Here's how the part is built. I have some questions about the finished solid (model axes, mm). Face numbers are marked on the shaded views. A direction names the side the tool comes from. Round coordinates to 2 decimals unless told otherwise and drop trailing zeros. Write each loop counter-clockwise with the first axis right and the second up, starting at its lowest first coordinate (ties: lowest second). Pieces come first, ordered by that corner, then holes. Notation, with made-up numbers: (69, 78.25) -> (89, 78.25) arc R28 cw to (89, 101.25) -> close; hole circle Ø4 at (-2, 20.25). An arc over 180 degrees is marked (long way). Put each result on its own line as item: value. Start each with the question number.
1. I need wall thicknesses on probe 1 along X at (y, z) = (5.75, 13); probe 2 along Z at (x, y) = (38.5, -3.75); probe 3 along Y at (x, z) = (0, 18.75). Which ranges of each line are inside material? Lowest first, please. Write a range as from..to.
2. We'd pull the mould along X, two halves only. Please class the marked faces 6, 7 and 8: +X half, -X half, draft (parallel to the pull), parting line (faces both ways), or undercut.
3. Which directions (+Z, -Z, +X, -X, +Y, -Y) give clear straight access to the entire face, cutting with the end or side of a thin tool? Please do the marked faces 1, 2, 3, 4 and 5.
4. Suppose I cut it at D-D (z = 6). Please give me the cut outline in (x, y), then the cut area to 3 significant figures.
5. Suppose I cut it at B-B (x = 38.5). Please give me the cut outline in (y, z), then the cut area to 3 significant figures.
6. For pin 1 (3 mm diameter, centred on y = 40, z = 13.5, fed in from +X); pin 2 (6 mm diameter, centred on x = -27.5, y = 18.5, fed in from -Z); pin 3 (12 mm diameter, centred on x = -24, z = 19.5, fed in from +Y); pin 4 (5 mm diameter, centred on y = 46, z = 13.5, fed in from -X), each with a flat end and sliding along its axis, tell me the tip position at first contact or that it passes through.
7. Suppose I cut it at C-C (y = 23.5). Please give me the cut outline in (x, z), then the cut area to 3 significant figures.
8. Suppose I cut it at A-A (z = 13). Please give me the cut outline in (x, y), then the cut area to 3 significant figures.
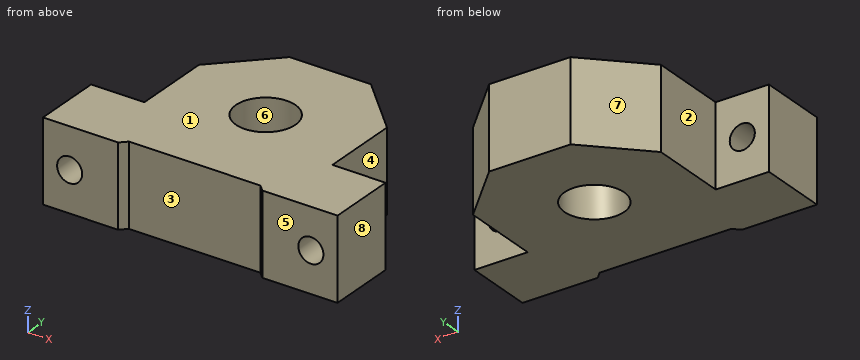
```python
from build123d import *

# Parameters (mm, degrees)
DODANIE_WYCI_GNI_CIE1_DEPTH = 26
SZKIC3_R                    = 9.5
WYTNIJ_WYCI_GNI_CIE1_DEPTH  = 26
SZKIC4_R                    = 4
WYTNIJ_WYCI_GNI_CIE2_DEPTH  = 22


with BuildPart() as part:
    # Szkic1 → Dodanie-wyciągnięcie1 (new body)
    with BuildSketch(Plane.XY):
        Polygon((-47, 11), (-30, 11), (-30, 36), (-13, 53), (13, 53), (30, 36), (30, 11), (47, 11), (47, -11), (23, -11), (21, -9), (-21, -9), (-23, -11), (-47, -11), align=None)
    extrude(amount=DODANIE_WYCI_GNI_CIE1_DEPTH)

    # Szkic3 → Wytnij-wyciągnięcie1 (cut)
    with BuildSketch(Plane(origin=(0, 0, 0), x_dir=(-1, 0, 0), z_dir=(0, 0, -1))):
        with Locations((0, 23.5)):
            Circle(SZKIC3_R)
    extrude(amount=-WYTNIJ_WYCI_GNI_CIE1_DEPTH, mode=Mode.SUBTRACT)

    # Szkic4 → Wytnij-wyciągnięcie2 (cut)
    with BuildSketch(Plane(origin=(0, 11, 0), x_dir=(1, 0, 0), z_dir=(0, 1, 0))):
        with Locations((38.5, -13)):
            Circle(SZKIC4_R)
        with Locations((-38.5, -13)):
            Circle(SZKIC4_R)
    extrude(amount=-WYTNIJ_WYCI_GNI_CIE2_DEPTH, mode=Mode.SUBTRACT)


solid = part.part
```
Verdict:
1. probe 1: x = -47..-42.5, -34.5..34.5, 42.5..47
1. probe 2: z = 0..9, 17..26
1. probe 3: y = -9..14, 33..53
2. face 6: undercut
2. face 7: -X half
2. face 8: +X half
3. face 1: +Z, +X, -X, +Y, -Y
3. face 2: +Z, -Z, -X, +Y
3. face 3: +Z, -Z, -Y
3. face 4: +Z, -Z, +X, +Y
3. face 5: +Z, -Z, +X, -X, -Y
4. outline: (-47, -11) -> (-23, -11) -> (-21, -9) -> (21, -9) -> (23, -11) -> (47, -11) -> (47, 11) -> (30, 11) -> (30, 36) -> (13, 53) -> (-13, 53) -> (-30, 36) -> (-30, 11) -> (-47, 11) -> close; hole circle Ø19 at (0, 23.5)
4. area: 3,930 mm^2
5. outline: (-11, 0) -> (11, 0) -> (11, 9) -> (-11, 9) -> close; (-11, 17) -> (11, 17) -> (11, 26) -> (-11, 26) -> close
5. area: 396 mm^2
6. pin 1: stops at x = 27.5
6. pin 2: stops at z = 0
6. pin 3: stops at y = 48
6. pin 4: stops at x = -22.5
7. outline: (-30, 0) -> (-9.5, 0) -> (-9.5, 26) -> (-30, 26) -> close; (9.5, 0) -> (30, 0) -> (30, 26) -> (9.5, 26) -> close
7. area: 1,070 mm^2
8. outline: (-47, -11) -> (-42.5, -11) -> (-42.5, 11) -> (-47, 11) -> close; (-34.5, -11) -> (-23, -11) -> (-21, -9) -> (21, -9) -> (23, -11) -> (34.5, -11) -> (34.5, 11) -> (30, 11) -> (30, 36) -> (13, 53) -> (-13, 53) -> (-30, 36) -> (-30, 11) -> (-34.5, 11) -> close; (42.5, -11) -> (47, -11) -> (47, 11) -> (42.5, 11) -> close; hole circle Ø19 at (0, 23.5)
8. area: 3,580 mm^2
